Can you work these out from the drawing? Everything is in mm from the part's minimum corner. A direction names the side the tool comes from. Coordinates: 2 decimals unless noted, no trailing zeros. Loops run counter-clockwise (first coordinate to the right, second up) from the corner with the lowest first, then second, coordinate; pieces in that order, holes last. Notation, with made-up numbers: M 79,75.25 L 111,75.25 A13 ccw 111,79.25 Z; hole C 61,16.25 d6. An arc over 180 degrees is marked long. Write each question's results on one line, items separated by ' | '.
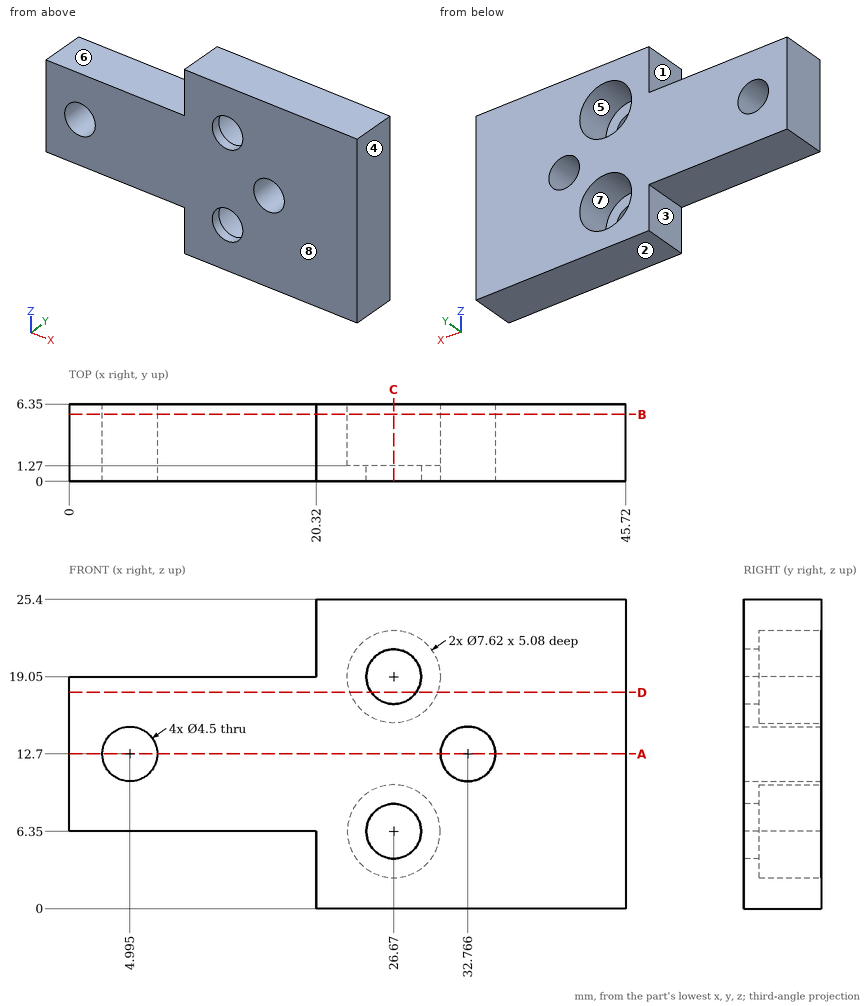
(1) If we mould it in two halves opening along Z, with no side actions, what happens to the marked faces 6, 7 and 8? For each: released by +Z, released by -Z, zero draft, split by the parting line, or undercut.
Reported:
face 6: released by +Z | face 7: undercut | face 8: zero draft
(2) Please list where these lines run through material, in increasing order: probe 1 along X at (y, z) = (2.5, 12.7) (3 decimals); probe 2 along Z at (x, y) = (26.67, 4.7); probe 3 along Z at (x, y) = (26.67, 0.35). Write a range as from..to.
Reported:
probe 1: x = 0..2.745, 7.245..30.516, 35.016..45.72 | probe 2: z = 0..2.54, 10.16..15.24, 22.86..25.4 | probe 3: z = 0..4.1, 8.6..16.8, 21.3..25.4
(3) Which directions (+Z, -Z, +X, -X, +Y, -Y) give clear straight access to the entire face, cutting with the end or side of a thin tool? Please do the marked faces 1, 2, 3, 4 and 5.
Reported:
face 1: +Z, -X, +Y, -Y | face 2: -Z, +X, -X, +Y, -Y | face 3: -Z, -X, +Y, -Y | face 4: +Z, -Z, +X, +Y, -Y | face 5: +Y
(4) Imagine slicing it at D-D, the plane z = 17.75. List the corners of the cut face in (x, y) for me.
Reported:
outline: M 0,0 L 24.83,0 L 24.83,1.27 L 23.09,1.27 L 23.09,6.35 L 0,6.35 Z; M 28.51,0 L 45.72,0 L 45.72,6.35 L 30.25,6.35 L 30.25,1.27 L 28.51,1.27 Z
(5) Will these pins go through, and if not, where does the flat tip stop? P1, Ø6, axis at x = 27.5, z = 18.5, coming from the +Y side; P2, Ø1.5, axis at y = 5, z = 4, coming from the -X side; P3, Ø6, axis at x = 26.67, z = 6.35, coming from the +Y side; P4, Ø1.9, axis at x = 10.5, y = 3, coming from the -Z side.
Reported:
P1: stops at y = 6.35 | P2: stops at x = 20.32 | P3: stops at y = 1.27 | P4: stops at z = 6.35
(6) Imagine slicing it at C-C, the plane x = 26.67. List the corners of the cut face in (y, z) for me.
Reported:
outline: M 0,0 L 6.35,0 L 6.35,2.54 L 1.27,2.54 L 1.27,4.1 L 0,4.1 Z; M 0,8.6 L 1.27,8.6 L 1.27,10.16 L 6.35,10.16 L 6.35,15.24 L 1.27,15.24 L 1.27,16.8 L 0,16.8 Z; M 0,21.3 L 1.27,21.3 L 1.27,22.86 L 6.35,22.86 L 6.35,25.4 L 0,25.4 Z
(7) Imagine slicing it at B-B, the plane y = 5.5. List the corners of the cut face in (x, z) for me (3 decimals), and give its area (3 significant figures).
Reported:
outline: M 0,6.35 L 20.32,6.35 L 20.32,0 L 45.72,0 L 45.72,25.4 L 20.32,25.4 L 20.32,19.05 L 0,19.05 Z; hole C 4.995,12.7 d4.5; hole C 26.67,6.35 d7.62; hole C 26.67,19.05 d7.62; hole C 32.766,12.7 d4.5 | area: 780 mm2
(8) Imagine slicing it at A-A, the plane z = 12.7. List the corners of the cut face in (x, y) for me (3 decimals), and give its area (3 significant figures).
Reported:
outline: M 0,0 L 2.745,0 L 2.745,6.35 L 0,6.35 Z; M 7.245,0 L 30.516,0 L 30.516,6.35 L 7.245,6.35 Z; M 35.016,0 L 45.72,0 L 45.72,6.35 L 35.016,6.35 Z | area: 233 mm2
